```python
from build123d import *

# Parameters (mm, degrees)
F0_W     = 50
F0_H     = 50
F0_R     = 1.5
F0_R_2   = 21.068216
F1_DEPTH = 8
F3_DEPTH = 100
F4_R     = 23.068216
F4_R_2   = 21.068216
F5_DEPTH = 80
F6_R     = 5


with BuildPart() as f1:
    # F0 (on Top) → F1 (new body)
    with BuildSketch(Plane.XY):
        Rectangle(F0_W, F0_H)
        with Locations((-20, -20)):
            Circle(F0_R, mode=Mode.SUBTRACT)
        with Locations((20, -20)):
            Circle(F0_R, mode=Mode.SUBTRACT)
        with Locations((-20, 20)):
            Circle(F0_R, mode=Mode.SUBTRACT)
        Circle(F0_R_2, mode=Mode.SUBTRACT)
        with Locations((20, 20)):
            Circle(F0_R, mode=Mode.SUBTRACT)
    extrude(amount=F1_DEPTH)

    # F2 (on face) → F3 (cut)
    with BuildSketch(Plane.XZ.offset(25)):
        with BuildLine():
            ThreePointArc((25, 6), (0, 3.249722), (-25, 6))
            Line((-25, 6), (-25, 0))
            Line((-25, 0), (25, 0))
            Line((25, 0), (25, 6))
        make_face()
    extrude(amount=-F3_DEPTH, mode=Mode.SUBTRACT)

    # F4 (on face) → F5 (join)
    with BuildSketch(Plane.XY.offset(8)):
        Circle(F4_R)
        Circle(F4_R_2, mode=Mode.SUBTRACT)
    extrude(amount=F5_DEPTH)

    # F6
    f6_edges = [f1.edges().sort_by_distance(p)[0] for p in [
        (25, -25, 7),
        (25, 25, 7),
        (-25, 25, 7),
        (-25, -25, 7),
    ]]
    fillet(f6_edges, radius=F6_R)


solid = f1.part
```
Model file for the job. Use its own axes, mm. A direction names the side the tool comes from. Round coordinates to 2 decimals unless told otherwise and drop trailing zeros. Loops run counter-clockwise (first coordinate to the right, second up) from the corner with the lowest first, then second, coordinate; pieces in that order, holes last. Notation, with made-up numbers: M 10.5,15 L 61.5,15 A6 ccw 61.5,24 Z; hole C 30.25,-8 d8. An arc over 180 degrees is marked long. Put each result on its own line as item: value. Start each with the question number.
Item 1: Mould opens along X. For faces 3 (the face through (-18.57, 20.45, 6.35)), 4 (the face through (0, 25, 6)), 5 (the face through (-18.57, -19.55, 6.35)), 6 (the face through (24, 23, 7)) say: released by +X, released by -X, zero draft, split by the parting line, or undercut.
Item 2: Cut at B-B (y = -12). List the corners of the cut face in (x, z), then the cut area to 3 significant figures.
Item 3: Drop flat-ended pins along their axis: P1, Ø2, axis at x = 19.5, z = 31, coming from the -Y side; P2, Ø3.5, axis at x = -20, y = 20, coming from the -Z side; P3, Ø12, axis at y = 16.5, z = 18, coming from the -X side. Give the stop position or say it passes through.
Item 4: Cut at C-C (z = 73.5). List the corners of the cut face in (x, y).
Item 5: Cut at A-A (x = 0). List the corners of the cut face in (y, z).
Item 6: 3-axis set-ups, long thin cutter, end or side, ignore diameter. For faces 1 (the face through (25, 0, 7)), 2 (the face through (-8, -22, 8)): which of +Z, -Z, +X, -X, +Y, -Y reach the whole face in a straight line?
Item 7: Drill centre lines: line 1 along Y through (x, z) = (0, 39); line 2 along Y through (x, z) = (7, 40.5); line 3 along X through (y, z) = (5, 72). Where is each one in solid material? Low to high.
Answer block:
1. face 3: undercut
1. face 4: zero draft
1. face 5: undercut
1. face 6: released by +X
2. outline: M -25,6 A115 ccw -17.32,4.56 L -17.32,88 L -19.7,88 L -19.7,8 L -25,8 Z; M 17.32,4.56 A115 ccw 25,6 L 25,8 L 19.7,8 L 19.7,88 L 17.32,88 Z
2. area: 424 mm2
3. P1: y = -13.78
3. P2: z = 4.71
3. P3: x = -20.54
4. outline: C 0,0 d46.14; hole C 0,0 d42.14
5. outline: M -25,3.25 L -21.07,3.25 L -21.07,88 L -23.07,88 L -23.07,8 L -25,8 Z; M 21.07,3.25 L 25,3.25 L 25,8 L 23.07,8 L 23.07,88 L 21.07,88 Z
6. face 1: +Z, -Z, +X, +Y, -Y
6. face 2: +Z
7. line 1: -23.07 to -21.07, 21.07 to 23.07
7. line 2: -21.98 to -19.87, 19.87 to 21.98
7. line 3: -22.52 to -20.47, 20.47 to 22.52
